CAD build for the part. Positions are in the model's coordinates, mm. Face numbers are marked on the shaded views. A direction names the side the tool comes from. Round coordinates to 2 decimals unless told otherwise and drop trailing zeros. Write each loop counter-clockwise with the first axis right and the second up, starting at its lowest first coordinate (ties: lowest second). Pieces come first, ordered by that corner, then holes. Notation, with made-up numbers: (-3.5, -7) -> (53.5, -7) arc R18 ccw to (53.5, 11) -> close; hole circle Ø1 at (43, 85.5). An arc over 180 degrees is marked (long way). Answer in a Markdown table with one row per item. Add a question column.
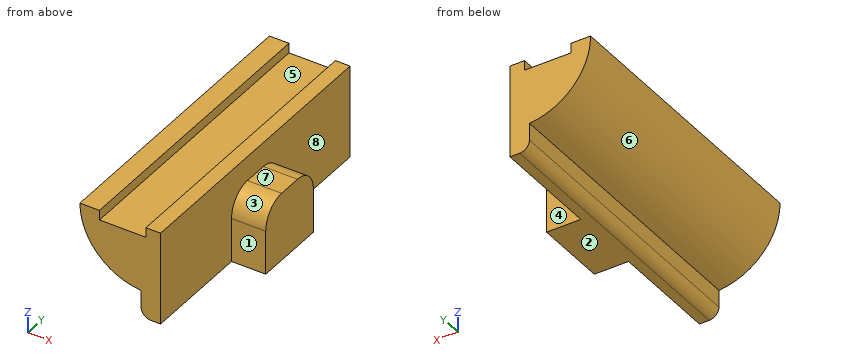
```python
from build123d import *

# Parameters (mm, degrees)
F1_DEPTH = 59.6
F2_R     = 2
F3_W     = 15
F3_H     = 14
F4_DEPTH = 7
F5_R     = 5


with BuildPart() as f1:
    # F0 (on Front) → F1 (new body)
    with BuildSketch(Plane.XZ):
        with BuildLine():
            Line((0, -9.5), (0, 7.5))
            Line((0, 7.5), (-9.5, 7.5))
            Line((-9.5, 7.5), (-9.5, 9.5))
            Line((-9.5, 9.5), (-13.5, 9.5))
            ThreePointArc((-13.5, 9.5), (-9.89512, 0.300815), (-1, -4))
            Line((-1, -4), (-1, -9.5))
            Line((-1, -9.5), (0, -9.5))
        make_face()
        Polygon((3, 9.5), (0, 9.5), (0, 7.5), (0, -9.5), (3, -9.5), align=None)
    extrude(amount=F1_DEPTH)

    # F2
    f2_edges = [f1.edges().sort_by_distance(p)[0] for p in [
        (-1, -29.8, -9.5),
    ]]
    fillet(f2_edges, radius=F2_R)

    # F3 (on face) → F4 (join)
    with BuildSketch(Plane.YZ.offset(3)):
        with Locations((-29.8, -2.5)):
            Rectangle(F3_W, F3_H)
    extrude(amount=F4_DEPTH)

    # F5
    f5_edges = [f1.edges().sort_by_distance(p)[0] for p in [
        (6.5, -37.3, 4.5),
        (6.5, -22.3, 4.5),
    ]]
    fillet(f5_edges, radius=F5_R)


solid = f1.part
```
Item 1: Saw through at D-D on y = -25.5. Give the cut face in (x, z), then the cut area to 3 significant figures.
Item 2: Saw through at C-C on z = 1.5. Give the cut face in (x, y).
Item 3: Pin check, flat tips, straight feed: pin 1 (3 mm diameter, centred on x = 0.5, y = -36.5, fed in from -Z); pin 2 (3 mm diameter, centred on y = -31.5, z = -6.5, fed in from -X); pin 3 (0.6 mm diameter, centred on y = -38, z = 8.5, fed in from +X); pin 4 (5 mm diameter, centred on x = -6.5, y = -43.5, fed in from +Z). Stop position of each tip, or through.
Item 4: Drill centre lines: probe 1 along Y at (x, z) = (8, -7.5); probe 2 along Z at (x, y) = (6.5, -29); probe 3 along X at (y, z) = (-49.5, -6). Where is each one in solid material? Low to high.
Item 5: Saw through at B-B on x = 4.5. Give the cut face in (y, z).
Item 6: Tool access for the marked faces 1, 2, 3 and 4: list every direction of +Z, -Z, +X, -X, +Y, -Y with a clear straight run to the whole face (end or side of a thin tool).
Item 7: Saw through at A-A on y = -39. Give the cut face in (x, z).
Item 8: Two-plate mould, pull along X, no slides. Class the marked faces 5, 6, 7 and 8: +X half, -X half, draft (parallel to the pull), parting line (faces both ways), or undercut.
Recorded:
| question | item | result |
|---|---|---|
| 1 | outline | (-13.5, 9.5) arc R13.54 ccw to (-1, -4) -> (-1, -7.5) arc R2 ccw to (1, -9.5) -> (10, -9.5) -> (10, 4.16) -> (3, 4.16) -> (3, 9.5) -> (0, 9.5) -> (0, 7.5) -> (-9.5, 7.5) -> (-9.5, 9.5) -> close |
| 1 | area | 282 mm2 |
| 2 | outline | (-10.88, -59.6) -> (3, -59.6) -> (3, -36.88) -> (10, -36.88) -> (10, -22.72) -> (3, -22.72) -> (3, 0) -> (-10.88, 0) -> close |
| 3 | pin 1 | z = -9.5 |
| 3 | pin 2 | x = -1 |
| 3 | pin 3 | x = 3 |
| 3 | pin 4 | z = 7.5 |
| 4 | probe 1 | -37.3 to -22.3 |
| 4 | probe 2 | -9.5 to 4.5 |
| 4 | probe 3 | -1 to 3 |
| 5 | outline | (-37.3, -9.5) -> (-22.3, -9.5) -> (-22.3, -0.5) arc R5 ccw to (-27.3, 4.5) -> (-32.3, 4.5) arc R5 ccw to (-37.3, -0.5) -> close |
| 6 | face 1 | +Z, -Z, +X, -Y |
| 6 | face 2 | -Z, +X, -X, +Y, -Y |
| 6 | face 3 | +Z, +X, -Y |
| 6 | face 4 | +Z, -Z, +X, +Y |
| 7 | outline | (-13.5, 9.5) arc R13.54 ccw to (-1, -4) -> (-1, -7.5) arc R2 ccw to (1, -9.5) -> (3, -9.5) -> (3, 9.5) -> (0, 9.5) -> (0, 7.5) -> (-9.5, 7.5) -> (-9.5, 9.5) -> close |
| 8 | face 5 | undercut |
| 8 | face 6 | -X half |
| 8 | face 7 | draft |
| 8 | face 8 | +X half |
